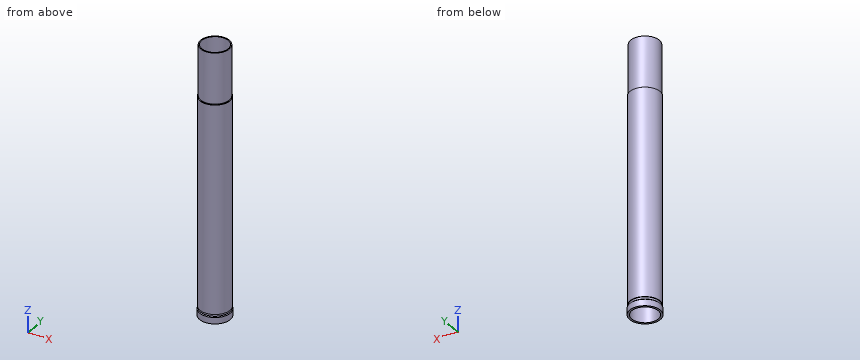
Autodesk Inventor part; units mm, degrees
ref_plane "YZ Plane" through (0, 0, 0) normal (1, 0, 0) x (0, 1, 0)
ref_plane "XZ Plane" through (0, 0, 0) normal (0, 1, 0) x (-1, 0, 0)
ref_plane "XY Plane" through (0, 0, 0) normal (0, 0, 1) x (1, 0, 0)
sketch "Skizze1" plane through (0, 0, 0) normal (0, 0, 1) x (1, 0, 0)
  circle A0 centre (0, 0) radius 13
  circle A1 centre (0, 0) radius 15
  dimension "d0" = 30
  dimension "d1" = 2
extrude "Extrusion1" add sketch "Skizze1" along normal blind 262
sketch "Skizze2" plane through (0, 0, 262) normal (0, 0, 1) x (1, 0, 0)
  circle A0 centre (0, 0) radius 15
  circle A1 centre (0, 0) radius 14.75
  dimension "d4" = 29.5
extrude "Extrusion2" cut sketch "Skizze2" against normal through all
sketch "Skizze3" plane through (0, 0, 0) normal (0, 0, -1) x (-1, 0, 0)
  circle A0 centre (0, 0) radius 14.75
  circle A1 centre (0, 0) radius 13
  circle A2 centre (0, 0) radius 15
  dimension "d7" = 30
extrude "Extrusion3" add sketch "Skizze3" against normal blind 9 contours A2
sketch "Skizze4" plane through (0, 0, 262) normal (0, 0, 1) x (1, 0, 0)
  circle A0 centre (0, 0) radius 14.75
  circle A1 centre (0, 0) radius 13
  circle A2 centre (0, 0) radius 14
  dimension "d10" = 28
extrude "Extrusion4" cut sketch "Skizze4" against normal blind 50 contours A0
sketch "Skizze5" plane through (0, 0, 0) normal (0, 1, 0) x (-1, 0, 0)
  line L0 (-15, 9) -> (15, 9)
  line L1 (15, 0) -> (-15, 0)
  line L2 (14.75, 9) -> (-14.75, 9)
  line L3 (15, 0) -> (15, 9)
  line L4 (13, 0) -> (13, 262)
  line L5 (14.75, 212) -> (14.75, 9)
  line L6 (15, 9) -> (14.25, 9)
  line L7 (14.25, 9) -> (14.25, 7)
  line L8 (14.25, 7) -> (15, 7)
  line L9 (15, 7) -> (15, 9)
  line L10 (21, 0) -> (-21, 0)
  line L11 (0, -50) -> (0, 300)
  point P0 (0, 0)
  point P1 (-9.75, 200)
  point P2 (9.75, 200)
  dimension "d13" = 2
  dimension "d14" = 28.5
revolve "Umdrehung1" cut sketch "Skizze5" angle 360 about axis through (0, 0, -10) along (0, 0, 1) contours L0 L3 L8 L7
chamfer "Fase1" distance 0.75 angle 45 1 edges at (15, 0, 7)
thread "Gewinde4"
fillet "Rundung1" radius 0.5 1 edges at (-14, 0, 212)
properties part number "13_0204_026"
Could you check a few things on this model? Use its own coordinates, in mm. Give positions to 0.01 mm unless a question says otherwise; leave off trailing zeros. Order: outer loops, then holes, each group sorted by start corner. A loop starts at its lowest first (then second) coordinate and runs counter-clockwise, first axis right, second up.
Q1. Suppose I cut it at C-C, the plane z = 74.5. Write out the boundary of the cut face in (x, y).
Q2. If I drill on line 1 along Y through (x, z) = (0, 157.5); line 2 along X through (y, z) = (-6.5, 183); line 3 along X through (y, z) = (-3, 217.5), over which ranges is the centre line in solid material (lowest first)?
Q3. Suppose I cut it at D-D, the plane z = 224.5. Write out the boundary of the cut face in (x, y), and give its area (3 significant figures).
Q4. I'm going to push flat-ended pins straight in: P1, Ø12, axis at x = 9.5, z = 162, coming from the +Y side; P2, Ø12, axis at x = -7.5, z = 196.5, coming from the -Y side; P3, Ø14.5, axis at x = 6, y = -1, coming from the +Z side; P4, Ø8, axis at y = 1, z = 58.5, coming from the +X side. Where does each tip first touch, or does it pass through?
Solution:
1. outline: circle Ø29.5 at (0, 0); hole circle Ø26 at (0, 0)
2. line 1: y = -14.75 to -13, 13 to 14.75
2. line 2: x = -13.24 to -11.26, 11.26 to 13.24
2. line 3: x = -13.67 to -12.65, 12.65 to 13.67
3. outline: circle Ø28 at (0, 0); hole circle Ø26 at (0, 0)
3. area: 84.8 mm2
4. P1: stops at y = 14.33
4. P2: stops at y = -14.67
4. P3: stops at z = 262
4. P4: stops at x = 14.75
